```python
from build123d import *


with BuildPart() as f1:
    # F0 (on Front) → F1 (revolve)
    with BuildSketch(Plane.XZ):
        with BuildLine():
            Line((0, 3.626402), (0, 0))
            Line((0, 0), (6.8, 0))
            Line((6.8, 0), (6.8, 3.3))
            Line((6.8, 3.3), (12.8, 3.3))
            Line((12.8, 3.3), (12.8, 5.1))
            Line((12.8, 5.1), (15.1, 5.1))
            Line((15.1, 5.1), (15.1, 6.7))
            Line((15.1, 6.7), (17, 6.7))
            Line((17, 6.7), (17, 8))
            Line((17, 8), (16.5, 9.5))
            Line((16.5, 9.5), (16.5, 15))
            Line((16.5, 15), (16.8, 16.552417))
            Line((16.8, 16.552417), (16.8, 20))
            Line((16.8, 20), (13.056557, 26.483833))
            Line((13.056557, 26.483833), (11.494917, 28.280295))
            ThreePointArc((11.494917, 28.280295), (9.794835, 29.549806), (7.721369, 30))
            Line((7.721369, 30), (7, 30))
            Line((7, 30), (5, 28))
            Line((5, 28), (3, 30))
            Line((3, 30), (2, 30))
            ThreePointArc((2, 30), (0.585786, 29.414214), (0, 28))
            Line((0, 28), (0, 24.78538))
            ThreePointArc((0, 24.78538), (0.138391, 24.054345), (0.534413, 23.424478))
            Line((0.534413, 23.424478), (10.988391, 12.166348))
            ThreePointArc((10.988391, 12.166348), (11.471216, 10.354122), (10.240762, 8.938755))
            Line((10.240762, 8.938755), (1.282042, 5.493093))
            ThreePointArc((1.282042, 5.493093), (0.351377, 4.758675), (0, 3.626402))
        make_face()
    revolve(axis=Axis((3.4, 0, 0), (-1, 0, 0)))


solid = f1.part
```
Here's how the part is built. I have some questions about the finished solid (model axes, mm). A direction names the side the tool comes from. Coordinates: 2 decimals unless noted, no trailing zeros. Order: outer loops, then holes, each group sorted by start corner. A loop starts at its lowest first (then second) coordinate and runs counter-clockwise, first axis right, second up. Notation, with made-up numbers: M -11.5,60.25 L 15.5,60.25 A20 ccw 15.5,73.25 Z; hole C 54,-20 d1. An arc over 180 degrees is marked long. Answer as a JSON object with one key per item and string values. Group by question number.
(1) Which directions (+Z, -Z, +X, -X, +Y, -Y) give clear straight access to the entire face, cutting with the end or side of a thin tool? Please do faces 5 (the face through (0, 0, 0)), 6 (the face through (16.063, 0.295, -6.694)).
(2) For pin 1 (5 mm diameter, centred on x = 12, y = -5, fed in from +Z); pin 2 (5 mm diameter, centred on y = -18, z = -2.5, fed in from -X); pin 3 (2 mm diameter, centred on x = 13, y = 12, fed in from +Z), each with a flat end and sliding along its axis, tell me the tip position at first contact or that it passes through.
(3) I need wall thicknesses on probe 1 along Z at (x, y) = (9.25, 2.5); probe 2 along Y at (x, z) = (9.5, 0); probe 3 along Y at (x, z) = (14.3, 0). Which ranges of each line are inside material? Lowest first, please.
(4) If we mould it in two halves opening along Z, with no side actions, what happens to faces 1 (the face through (16.5, -10, 0)), 2 (the face through (4.87, 8.45, 26.83)), 3 (the face through (16.8, 15, 8)), 4 (the face through (12.8, -1.1, -3.3))? For each: released by +Z, released by -Z, zero draft, split by the parting line, or undercut.
(5) Suppose I cut it at A-A, the plane x = 9.5. Please give me the cut outline in (y, z), then the cut area to 3 significant figures.
Values found:
{
 "1": {"face 5": "+Z, -Z, -X, +Y, -Y", "face 6": "+X"},
 "2": {"pin 1": "stops at z = 29.32", "pin 2": "stops at x = 3.09", "pin 3": "stops at z = 25.05"},
 "3": {"probe 1": "z = -29.66 to -13.81, -8.18 to -2.15, 2.15 to 8.18, 13.81 to 29.66", "probe 2": "y = -29.67 to -13.77, -8.65 to -3.3, 3.3 to 8.65, 13.77 to 29.67", "probe 3": "y = -24.33 to -5.1, 5.1 to 24.33"},
 "4": {"face 1": "undercut", "face 2": "split by the parting line", "face 3": "zero draft", "face 4": "undercut"},
 "5": {"outline": "C 0,0 d59.35; C 0,0 d17.31; hole C 0,0 d27.54; hole C 0,0 d6.6", "area": "2,370 mm^2"}
}
